```python
from build123d import *

# Parameters (mm, degrees)
SKETCH1_R           = 9.9
SKETCH1_R_2         = 4.03
BOSS_EXTRUDE1_DEPTH = 6.35
SKETCH2_W           = 6.15
SKETCH2_H           = 3.189666584
BOSS_EXTRUDE2_DEPTH = 6.35
FILLET2_R           = 1


with BuildPart() as part:
    # Sketch1 → Boss-Extrude1 (new body)
    with BuildSketch(Plane(origin=(0, 0, 0), x_dir=(1, 0, 0), z_dir=(0, 1, 0))):
        Circle(SKETCH1_R)
        Circle(SKETCH1_R_2, mode=Mode.SUBTRACT)
    extrude(amount=BOSS_EXTRUDE1_DEPTH)

    # Sketch2 → Boss-Extrude2 (add, through all)
    with BuildSketch(Plane.XZ):
        with Locations((0, 11.005166708)):
            Rectangle(SKETCH2_W, SKETCH2_H)
        with Locations((0, -11.005166708)):
            Rectangle(SKETCH2_W, SKETCH2_H)
    extrude(amount=-BOSS_EXTRUDE2_DEPTH)

    # Fillet2
    fillet2_edges = [part.edges().sort_by_distance(p)[0] for p in [
        (-3.075, 3.175, 9.410333416),
        (-3.075, 3.175, 12.6),
        (3.075, 3.175, 12.6),
        (3.075, 3.175, 9.410333416),
        (-3.075, 3.175, -12.6),
        (-3.075, 3.175, -9.410333416),
        (3.075, 3.175, -9.410333416),
        (3.075, 3.175, -12.6),
    ]]
    fillet(fillet2_edges, radius=FILLET2_R)


solid = part.part
```
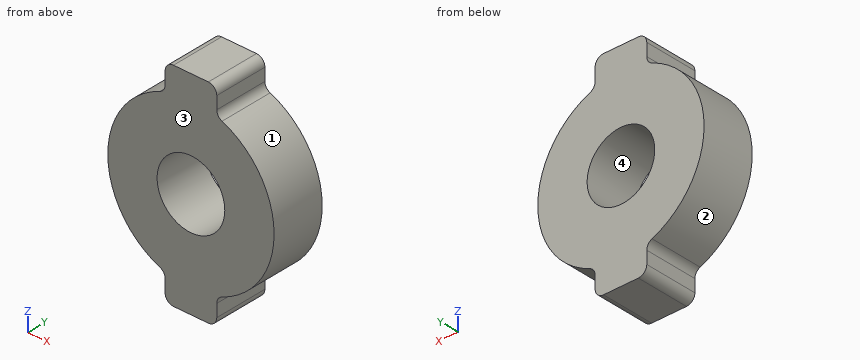
Here's how the part is built. I have some questions about the finished solid (model axes, mm). Face numbers are marked on the shaded views. Round coordinates to 2 decimals unless told otherwise and drop trailing zeros. Write each loop counter-clockwise with the first axis right and the second up, starting at its lowest first coordinate (ties: lowest second). Pieces come first, ordered by that corner, then holes. Notation, with made-up numbers: M -9,-36.5 L 3,-36.5 A14 cw 3,-10.5 Z; hole C -40,15.25 d8. An arc over 180 degrees is marked long. Answer as CSV lines item,"result". Start each with the question number.
1. Suppose I cut it at B-B on y = 5.75. Write out the boundary of the cut face in (x, z) (3 decimals), then the cut area to 3 significant figures.
2. Suppose I cut it at C-C on x = 0. Write out the boundary of the cut face in (y, z), then the cut area to 3 significant figures.
3. I need wall thicknesses on probe 1 along Z at (x, y) = (0, 4); probe 2 along X at (y, z) = (1, -2.75); probe 3 along X at (y, z) = (3.75, 11) (3 decimals). Which ranges of each line are inside material? Lowest first, please.
4. Suppose I cut it at D-D on z = 10.5. Write out the boundary of the cut face in (x, y) (3 decimals), then the cut area to 3 significant figures.
5. I'm going to push flat-ended pins straight in: pin 1 Ø2 at (x, y) = (-5, 1) entering from -Z; pin 2 Ø1.5 at (y, z) = (1.5, 7) entering from -X; pin 3 Ø1.2 at (y, z) = (2, -10.5) entering from -X. Where does each tip first touch, or does it pass through?
6. Suppose I cut it at A-A on z = 0. Write out the boundary of the cut face in (x, y).
7. Thinking about a two-plate mould opening in X: for the marked faces 1, 2, 3 and 4, which applies, released by +X, released by -X, zero draft, split by the parting line, or undercut?
Check result:
1,outline,"M -3.701,-9.182 A1 cw -3.075,-10.11 L -3.075,-11.6 A1 ccw -2.075,-12.6 L 2.075,-12.6 A1 ccw 3.075,-11.6 L 3.075,-10.11 A1 cw 3.701,-9.182 A9.9 ccw 3.701,9.182 A1 cw 3.075,10.11 L 3.075,11.6 A1 ccw 2.075,12.6 L -2.075,12.6 A1 ccw -3.075,11.6 L -3.075,10.11 A1 cw -3.701,9.182 A9.9 ccw Z; hole C 0,0 d8.06"
1,area,"292 mm2"
2,outline,"M 0,-12.6 L 6.35,-12.6 L 6.35,-4.03 L 0,-4.03 Z; M 0,4.03 L 6.35,4.03 L 6.35,12.6 L 0,12.6 Z"
2,area,"109 mm2"
3,probe 1,"z = -12.6 to -4.03, 4.03 to 12.6"
3,probe 2,"x = -9.51 to -2.95, 2.95 to 9.51"
3,probe 3,"x = -3.075 to 3.075"
4,outline,"M -3.075,0 L 3.075,0 L 3.075,6.35 L -3.075,6.35 Z"
4,area,"39.1 mm2"
5,pin 1,"stops at z = -9.06"
5,pin 2,"stops at x = -7.68"
5,pin 3,"stops at x = -3.1"
6,outline,"M -9.9,0 L -4.03,0 L -4.03,6.35 L -9.9,6.35 Z; M 4.03,0 L 9.9,0 L 9.9,6.35 L 4.03,6.35 Z"
7,face 1,"released by +X"
7,face 2,"released by -X"
7,face 3,"zero draft"
7,face 4,"undercut"
